```python
from build123d import *

# Parameters (mm, degrees)
SKETCH_1_W          = 105
SKETCH_1_H          = 35
SKETCH_1_R          = 1.75
EXTRUDE_1_DEPTH     = 3
SKETCH_3_W          = 24
SKETCH_3_H          = 35
EXTRUDE_2_DEPTH     = 3
SKETCH_4_W          = 95
SKETCH_4_H          = 135
EXTRUDE_3_DEPTH     = 3
SKETCH_2_R          = 1.65
CUT_EXTRUDE_1_DEPTH = 172.052623482


with BuildPart() as part:
    # 草图1 → 凸台-拉伸1 (new body)
    with BuildSketch(Plane.XY):
        with Locations((52.5, -17.5)):
            Rectangle(SKETCH_1_W, SKETCH_1_H)
        with Locations((19, -7)):
            Circle(SKETCH_1_R, mode=Mode.SUBTRACT)
        with Locations((10, -16)):
            Circle(SKETCH_1_R, mode=Mode.SUBTRACT)
        with Locations((19, -25)):
            Circle(SKETCH_1_R, mode=Mode.SUBTRACT)
        with Locations((28, -16)):
            Circle(SKETCH_1_R, mode=Mode.SUBTRACT)
    extrude(amount=EXTRUDE_1_DEPTH)

    # 草图3 → 凸台-拉伸2 (add)
    with BuildSketch(Plane.XY.offset(3)):
        with Locations((-12, -17.5)):
            Rectangle(SKETCH_3_W, SKETCH_3_H)
    extrude(amount=-EXTRUDE_2_DEPTH)

    # 草图4 → 凸台-拉伸3 (add)
    with BuildSketch(Plane.XY.offset(3)):
        with Locations((30.5, 67.5)):
            Rectangle(SKETCH_4_W, SKETCH_4_H)
    extrude(amount=-EXTRUDE_3_DEPTH)

    # 草图2 → 切除-拉伸1 (cut, through all)
    with BuildSketch(Plane.XY.offset(3)):
        with Locations((47, -3)):
            Circle(SKETCH_2_R)
        with Locations((59, -3)):
            Circle(SKETCH_2_R)
        with Locations((47, 11)):
            Circle(SKETCH_2_R)
        with Locations((59, 11)):
            Circle(SKETCH_2_R)
        with Locations((71, 11)):
            Circle(SKETCH_2_R)
        with Locations((35, 11)):
            Circle(SKETCH_2_R)
        with Locations((35, 1)):
            Circle(SKETCH_2_R)
        with Locations((71, 1)):
            Circle(SKETCH_2_R)
        with Locations((47, -17)):
            Circle(SKETCH_2_R)
        with Locations((59, -17)):
            Circle(SKETCH_2_R)
    extrude(amount=-CUT_EXTRUDE_1_DEPTH, mode=Mode.SUBTRACT)


solid = part.part
```
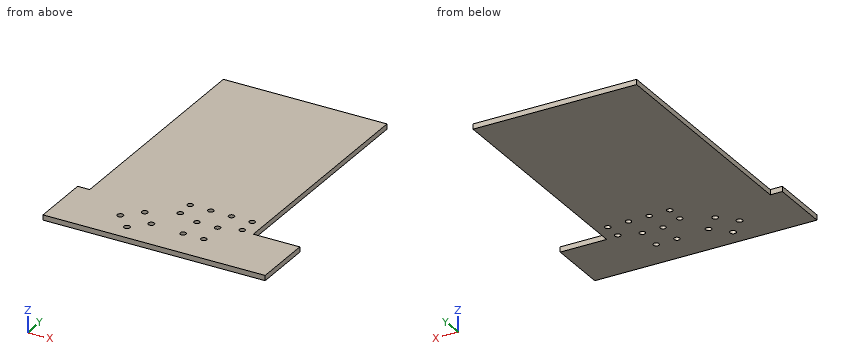
Verification items for the finished model (mm, model axes). Give positions to 0.01 mm unless a question says otherwise; leave off trailing zeros. Order: outer loops, then holes, each group sorted by start corner. A loop starts at its lowest first (then second) coordinate and runs counter-clockwise, first axis right, second up. Notation, with made-up numbers: M -27.75,67.25 L -10.75,67.25 A16 ccw -10.75,73.25 Z; hole C 56.5,86.25 d5. An arc over 180 degrees is marked long. Return JSON: item names as keys, results as strings. Group by question number.
1) Section check D-D on x = 88. Record the cut outline in (y, z), and give its area (3 significant figures).
2) Section check B-B on x = 28. Record the cut outline in (y, z).
3) Section check C-C on y = -25. Record the cut outline in (x, z), and give its area (4 significant figures).
4) Section check A-A on z = 1.55. Give the number of separate pieces and of enclosed holes in the cut face, and give its area (3 significant figures).
5) Go/stop test with flat-tipped pins: pin 1 Ø3 at (x, y) = (35, 1) entering from -Z; pin 2 Ø1.5 at (y, z) = (93, 1) entering from +X. Record where each tip stops, or that it passes through.
6) Scan lines: line 1 (Y direction, x = 47, z = 2.3); line 2 (Y direction, x = 35, z = 2.05); line 3 (Y direction, x = 28, z = 1.85). Record each from-to range of solid material in increasing order.
Answer block:
{
 "1": {"outline": "M -35,0 L 0,0 L 0,3 L -35,3 Z", "area": "105 mm^2"},
 "2": {"outline": "M -35,0 L -17.75,0 L -17.75,3 L -35,3 Z; M -14.25,0 L 135,0 L 135,3 L -14.25,3 Z"},
 "3": {"outline": "M -24,0 L 17.25,0 L 17.25,3 L -24,3 Z; M 20.75,0 L 105,0 L 105,3 L 20.75,3 Z", "area": "376.5 mm^2"},
 "4": {"separate pieces": "1", "enclosed holes": "14", "area": "17,200 mm^2"},
 "5": {"pin 1": "passes through", "pin 2": "stops at x = 78"},
 "6": {"line 1": "y = -35 to -18.65, -15.35 to -4.65, -1.35 to 9.35, 12.65 to 135", "line 2": "y = -35 to -0.65, 2.65 to 9.35, 12.65 to 135", "line 3": "y = -35 to -17.75, -14.25 to 135"}
}
